CAD build for the part. Positions are in the model's coordinates, mm. Face numbers are marked on the shaded views. A direction names the side the tool comes from. Round coordinates to 2 decimals unless told otherwise and drop trailing zeros. Loops run counter-clockwise (first coordinate to the right, second up) from the corner with the lowest first, then second, coordinate; pieces in that order, holes last.
```python
from build123d import *

# Parameters (mm, degrees)
SKETCH2_W           = 160
SKETCH2_H           = 50
BOSS_EXTRUDE1_DEPTH = 60
CUT_EXTRUDE1_DEPTH  = 61
SKETCH4_W           = 77
SKETCH4_H           = 36
CUT_EXTRUDE3_DEPTH  = 61
SKETCH9_W           = 77
SKETCH9_H           = 21
BOSS_EXTRUDE4_DEPTH = 30


with BuildPart() as part:
    # Sketch2 → Boss-Extrude1 (new body)
    with BuildSketch(Plane.XY):
        with Locations((21.725, 25)):
            Rectangle(SKETCH2_W, SKETCH2_H)
    extrude(amount=BOSS_EXTRUDE1_DEPTH)

    # Sketch3 → Cut-Extrude1 (cut, through all)
    with BuildSketch(Plane.XY.offset(60)):
        Polygon((-39.377928434, 50), (-26.275, 14), (-3.275, 14), (-3.275, 50), align=None)
    extrude(amount=-CUT_EXTRUDE1_DEPTH, mode=Mode.SUBTRACT)

    # Sketch4 → Cut-Extrude3 (cut, through all)
    with BuildSketch(Plane.XY.offset(60)):
        with Locations((43.225, 32)):
            Rectangle(SKETCH4_W, SKETCH4_H)
    extrude(amount=-CUT_EXTRUDE3_DEPTH, mode=Mode.SUBTRACT)

    # Sketch9 → Boss-Extrude4 (add)
    with BuildSketch(Plane(origin=(0, 14, 0), x_dir=(1, 0, 0), z_dir=(0, 1, 0))):
        with Locations((43.225, -30)):
            Rectangle(SKETCH9_W, SKETCH9_H)
    extrude(amount=BOSS_EXTRUDE4_DEPTH)


solid = part.part
```
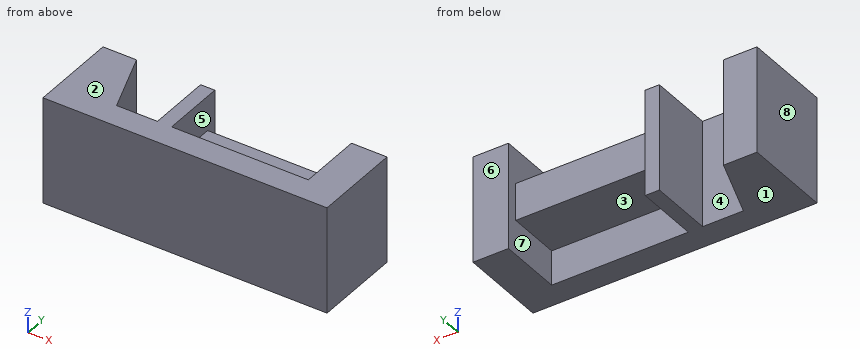
Item 1: Flat gauge pins, fed straight in: P1, Ø15.5, axis at x = 54, z = 13.5, coming from the +Y side; P2, Ø2, axis at x = -9.5, y = 16.5, coming from the +Z side; P3, Ø6, axis at x = 34, z = 47.5, coming from the +Y side; P4, Ø15, axis at x = 51.5, y = 36.5, coming from the -Z side. Where does each tip first touch, or does it go through?
Answers follow:
P1: stops at y = 44
P2: passes through
P3: stops at y = 14
P4: stops at z = 19.5
Item 2: Two-plate mould, pull along X, no slides. Class the marked faces 6, 7 and 8: released by +X, released by -X, zero draft, split by the parting line, or undercut.
Answers follow:
face 6: zero draft
face 7: undercut
face 8: released by -X
Item 3: Cut at C-C, the plane x = 28. Give the cut face in (y, z), plus the area to 3 significant figures.
Answers follow:
outline: (0, 0) - (14, 0) - (14, 19.5) - (44, 19.5) - (44, 40.5) - (14, 40.5) - (14, 60) - (0, 60) - close
area: 1,470 mm2
Item 4: Cut at A-A, the plane y = 39.5. Give the cut face in (x, z) (3 decimals).
Answers follow:
outline: (-58.275, 0) - (-35.556, 0) - (-35.556, 60) - (-58.275, 60) - close; (-3.275, 0) - (4.725, 0) - (4.725, 19.5) - (81.725, 19.5) - (81.725, 0) - (101.725, 0) - (101.725, 60) - (81.725, 60) - (81.725, 40.5) - (4.725, 40.5) - (4.725, 60) - (-3.275, 60) - close
Item 5: Cut at D-D, the plane y = 25. Give the cut face in (x, z) (3 decimals).
Answers follow:
outline: (-58.275, 0) - (-30.279, 0) - (-30.279, 60) - (-58.275, 60) - close; (-3.275, 0) - (4.725, 0) - (4.725, 19.5) - (81.725, 19.5) - (81.725, 0) - (101.725, 0) - (101.725, 60) - (81.725, 60) - (81.725, 40.5) - (4.725, 40.5) - (4.725, 60) - (-3.275, 60) - close
Item 6: Probe line 1 (X direction, y = 25.5, z = 46) (3 decimals); line 2 (X direction, y = 22, z = 48) (3 decimals); line 3 (Y direction, x = -9.5, z = 12). List the from-to ranges inside material, lowest first.
Answers follow:
line 1: x = -58.275 to -30.461, -3.275 to 4.725, 81.725 to 101.725
line 2: x = -58.275 to -29.187, -3.275 to 4.725, 81.725 to 101.725
line 3: y = 0 to 14
Item 7: 3-axis set-ups, long thin cutter, end or side, ignore diameter. For the marked faces 1, 2, 3, 4 and 5: which of +Z, -Z, +X, -X, +Y, -Y reach the whole face in a straight line?
Answers follow:
face 1: -Z, +X, -X, +Y, -Y
face 2: +Z, +X, -X, +Y, -Y
face 3: -Z, +Y
face 4: +Z, -Z, +Y
face 5: +Y
Item 8: Cut at B-B, the plane z = 56. Give the cut face in (x, y) (3 decimals), plus the area to 3 significant figures.
Answers follow:
outline: (-58.275, 0) - (101.725, 0) - (101.725, 50) - (81.725, 50) - (81.725, 14) - (4.725, 14) - (4.725, 50) - (-3.275, 50) - (-3.275, 14) - (-26.275, 14) - (-39.378, 50) - (-58.275, 50) - close
area: 4,160 mm2
